```python
from build123d import *

# Parameters (mm, degrees)
SKETCH2_W               = 41.91
SKETCH2_H               = 190.436
BOSS_EXTRUDE1_DEPTH     = 6.35
SKETCH3_R               = 3.3
CUT_EXTRUDE1_DEPTH      = 478.183864302
SKETCH4_W               = 10.033
SKETCH4_H               = 6.858
CUT_EXTRUDE2_DEPTH      = 474.191260281
CUT_EXTRUDE3_DEPTH      = 474.191260281
CUT_EXTRUDE3_DEPTH_BACK = 474.191260281
SKETCH5_R               = 3.3


with BuildPart() as part:
    # Sketch2 → Boss-Extrude1 (new body)
    with BuildSketch(Plane.XY):
        with Locations((-327.245441571, 231.003658294)):
            Rectangle(SKETCH2_W, SKETCH2_H)
    extrude(amount=BOSS_EXTRUDE1_DEPTH)

    # Sketch3 → Cut-Extrude1 (cut, through all)
    with BuildSketch(Plane.XY.offset(6.35)):
        Polygon((-314.418441571, 195.840658294), (-314.418441571, 203.079658294), (-342.708441633, 203.079658294), (-342.708441633, 257.927658294), (-314.418441571, 257.927658294), (-314.418441571, 265.166658294), (-342.708441633, 265.166658294), (-342.708441633, 321.014658294), (-314.418441571, 321.014658294), (-314.418441571, 326.221658294), (-348.200441571, 326.221658294), (-348.200441571, 135.785658294), (-314.418441571, 135.785658294), (-314.418441571, 140.992658294), (-342.708441633, 140.992658294), (-342.708441633, 195.840658294), align=None)
        with Locations((-332.325441571, 294.535658294)):
            Circle(SKETCH3_R)
        with Locations((-332.325441571, 231.035658294)):
            Circle(SKETCH3_R)
        with Locations((-332.325441571, 167.535658294)):
            Circle(SKETCH3_R)
    extrude(amount=-CUT_EXTRUDE1_DEPTH, mode=Mode.SUBTRACT)

    # Sketch4 → Cut-Extrude2 (cut, through all)
    with BuildSketch(Plane.XY.offset(6.35)):
        with Locations((-318.564971808, 144.167658294)):
            Rectangle(SKETCH4_W, SKETCH4_H)
        with Locations((-318.564971808, 192.656258294)):
            Rectangle(SKETCH4_W, SKETCH4_H)
        with Locations((-318.564971808, 206.245258294)):
            Rectangle(SKETCH4_W, SKETCH4_H)
        with Locations((-318.564971808, 254.759258294)):
            Rectangle(SKETCH4_W, SKETCH4_H)
        with Locations((-318.564971808, 268.348258294)):
            Rectangle(SKETCH4_W, SKETCH4_H)
        with Locations((-318.564971808, 317.852858294)):
            Rectangle(SKETCH4_W, SKETCH4_H)
    extrude(amount=-CUT_EXTRUDE2_DEPTH, mode=Mode.SUBTRACT)

    # Sketch5 → Cut-Extrude3 (cut, two sides: drawn at the far end of the back side and taken through both)
    with BuildSketch(Plane.XY.offset(6.35).offset(-CUT_EXTRUDE3_DEPTH_BACK)):
        Polygon((-314.418441571, 264.919258294), (-314.418441571, 262.785658294), (-306.290441571, 262.785658294), (-306.290441571, 326.221658294), (-314.418441571, 326.221658294), (-314.418441571, 321.281858294), (-313.548471808, 321.281858294), (-313.548471808, 314.423858294), (-323.581471808, 314.423858294), (-323.581471808, 321.014658294), (-342.708441633, 321.014658294), (-342.708441633, 265.166658294), (-323.581471808, 265.166658294), (-323.581471808, 271.777258294), (-313.548471808, 271.777258294), (-313.548471808, 264.919258294), align=None)
        with Locations((-332.325441571, 294.535658294)):
            Circle(SKETCH5_R, mode=Mode.SUBTRACT)
    extrude(amount=CUT_EXTRUDE3_DEPTH + CUT_EXTRUDE3_DEPTH_BACK, mode=Mode.SUBTRACT)


solid = part.part
```
Build history of the part. All positions in model axes, mm. A direction names the side the tool comes from. Give positions to 0.01 mm unless a question says otherwise; leave off trailing zeros. Loops run counter-clockwise (first coordinate to the right, second up) from the corner with the lowest first, then second, coordinate; pieces in that order, holes last. Notation, with made-up numbers: (9, -27.5) - (47, -27.5) arc R9 cw to (47, -11.5) - close; hole circle Ø8 at (76, 63). An arc over 180 degrees is marked (long way). Use a Markdown table: item, result.
(1) Band-saw the part on B-B (z = 3.75). Give the number of separate pieces and of enclosed holes in the cut face, and give its area (3 significant figures).
Taken from the geometry:
| item | result |
|---|---|
| separate pieces | 1 |
| enclosed holes | 2 |
| area | 3,800 mm2 |
(2) Pull direction Y, two halves, no side cores. Call faces 5 (the face through (-310, 262.786, 3)), 6 (the face through (-323.581, 144, 3)), 7 (the face through (-313.548, 206, 3)): +Y half, -Y half, draft (parallel to the pull), parting line (faces both ways), or undercut.
Taken from the geometry:
| item | result |
|---|---|
| face 5 | +Y half |
| face 6 | draft |
| face 7 | undercut |
(3) Drop flat-ended pins along their axis: pin 1 Ø3 at (x, z) = (-319.5, 2) entering from +Y; pin 2 Ø3 at (x, z) = (-336, 5) entering from +Y. Give the stop position or say it passes through.
Taken from the geometry:
| item | result |
|---|---|
| pin 1 | y = 251.33 |
| pin 2 | y = 257.93 |
(4) Band-saw the part on C-C (x = -319). Give the cut face in (y, z), and give its area (3 significant figures).
Taken from the geometry:
| item | result |
|---|---|
| outline | (147.6, 0) - (189.23, 0) - (189.23, 6.35) - (147.6, 6.35) - close; (209.67, 0) - (251.33, 0) - (251.33, 6.35) - (209.67, 6.35) - close |
| area | 529 mm2 |
(5) Which spindle directions (+Z, -Z, +X, -X, +Y, -Y) get a long thin tool onto all of the face, cutting with end or side? Do faces 1 (the face through (-333, 257.928, 3)), 2 (the face through (-313.548, 193, 3)), 3 (the face through (-323.581, 255, 3)), 4 (the face through (-314.418, 199, 3)). Say none if no direction does.
Taken from the geometry:
| item | result |
|---|---|
| face 1 | +Z, -Z, -X, +Y |
| face 2 | +Z, -Z |
| face 3 | +Z, -Z, +Y |
| face 4 | +Z, -Z, -X |
(6) Band-saw the part on A-A (x = -340). Give the cut face in (y, z).
Taken from the geometry:
| item | result |
|---|---|
| outline | (140.99, 0) - (195.84, 0) - (195.84, 6.35) - (140.99, 6.35) - close; (203.08, 0) - (257.93, 0) - (257.93, 6.35) - (203.08, 6.35) - close |
(7) Wall check: line 1 along Y through (x, z) = (-316, 0.75); line 2 along Y through (x, z) = (-336.5, 2.5); line 3 along X through (y, z) = (196.5, 4). Give the ranges that are in metal, low to high.
Taken from the geometry:
| item | result |
|---|---|
| line 1 | 147.6 to 189.23, 209.67 to 251.33 |
| line 2 | 140.99 to 195.84, 203.08 to 257.93 |
| line 3 | -314.42 to -306.29 |
